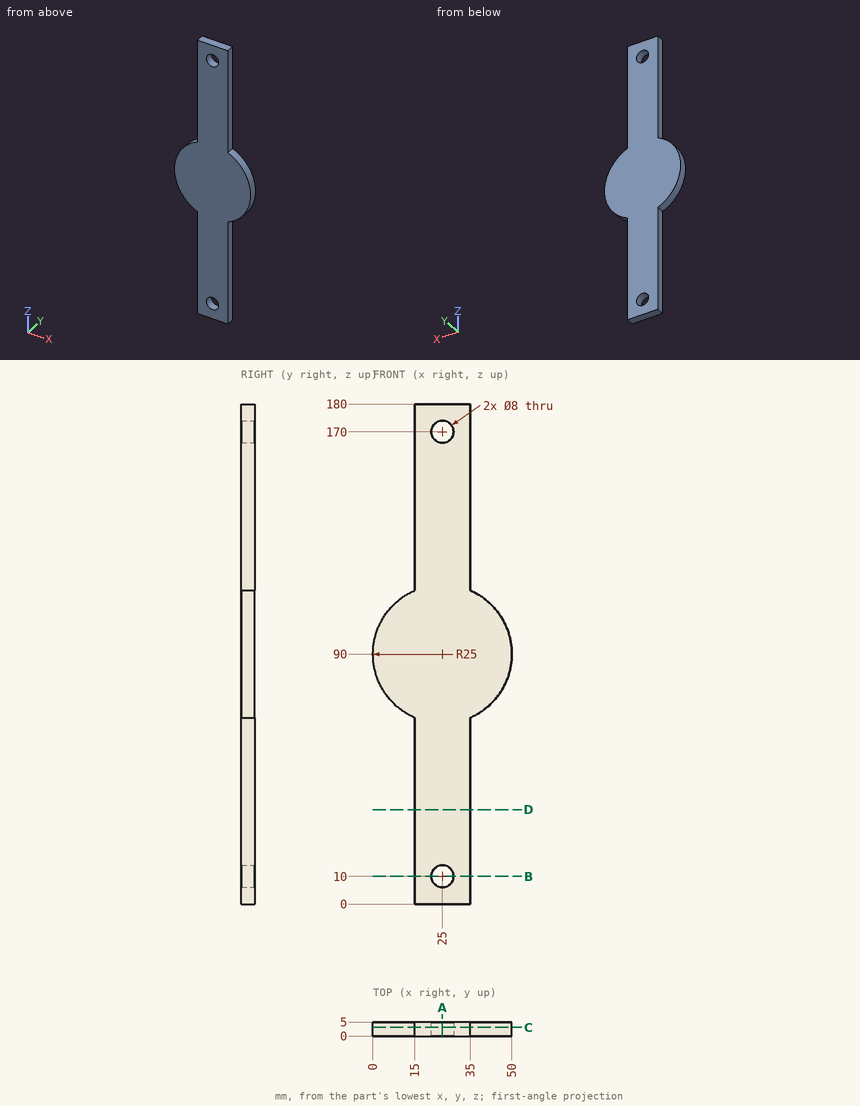
Answer from the drawing. Dimensions are ordinates in mm from the lowest x, y and z of the part. Give positions to 0.01 mm unless a question says otherwise; leave off trailing zeros. Loops run counter-clockwise (first coordinate to the right, second up) from the corner with the lowest first, then second, coordinate; pieces in that order, holes last.
Item 1: Each of these flat-tipped pins is pushed along its axis until it touches: pin 1 Ø3 at (x, z) = (14.5, 19) entering from +Y; pin 2 Ø6 at (x, z) = (39.5, 158.5) entering from +Y (3 decimals); pin 3 Ø2 at (y, z) = (1.5, 107) entering from +X; pin 4 Ø2.5 at (y, z) = (2, 43) entering from -X. Where does it stop, or does it pass through?
Item 2: The part is cut by section A-A (x = 25). Write down the section's boundary in (y, z).
Item 3: The part is cut by section B-B (z = 10). Write down the section's boundary in (x, y), and give its area (3 significant figures).
Item 4: The part is cut by section C-C (y = 3.1). Write down the section's boundary in (x, z).
Item 5: Find the intervals of material crossed by line 1 along Z through (x, y) = (25, 2.55); line 2 along X through (y, z) = (1.85, 170); line 3 along Z through (x, y) = (27, 3.7), in increasing order.
Item 6: The part is cut by section D-D (z = 34). Write down the section's boundary in (x, y), and give its area (3 significant figures).
Taken from the geometry:
1. pin 1: stops at y = 5
1. pin 2: passes through
1. pin 3: stops at x = 44.21
1. pin 4: stops at x = 15
2. outline: (0, 0) - (5, 0) - (5, 6) - (0, 6) - close; (0, 14) - (5, 14) - (5, 166) - (0, 166) - close; (0, 174) - (5, 174) - (5, 180) - (0, 180) - close
3. outline: (15, 0) - (21, 0) - (21, 5) - (15, 5) - close; (29, 0) - (35, 0) - (35, 5) - (29, 5) - close
3. area: 60.0 mm2
4. outline: (15, 0) - (35, 0) - (35, 67.09) arc R25 ccw to (35, 112.91) - (35, 180) - (15, 180) - (15, 112.91) arc R25 ccw to (15, 67.09) - close; hole circle Ø8 at (25, 10); hole circle Ø8 at (25, 170)
5. line 1: z = 0 to 6, 14 to 166, 174 to 180
5. line 2: x = 15 to 21, 29 to 35
5. line 3: z = 0 to 6.54, 13.46 to 166.54, 173.46 to 180
6. outline: (15, 0) - (35, 0) - (35, 5) - (15, 5) - close
6. area: 100 mm2
